```python
from build123d import *

# Parameters (mm, degrees)
SKETCH1_R           = 28.575
BOSS_EXTRUDE1_DEPTH = 22.225
SKETCH3_R           = 11.1125
BOSS_EXTRUDE2_DEPTH = 25.4
SKETCH4_R           = 22.225
CUT_EXTRUDE1_DEPTH  = 12.7
CUT_EXTRUDE2_DEPTH  = 23.225


with BuildPart() as part:
    # Sketch1 → Boss-Extrude1 (new body)
    with BuildSketch(Plane(origin=(0, 0, 0), x_dir=(1, 0, 0), z_dir=(0, 1, 0))):
        with BuildLine():
            Line((-69.85, 0), (69.85, 0))
            ThreePointArc((69.85, 0), (67.980720293, 10.733361765), (62.592988676, 20.202871225))
            ThreePointArc((62.592988676, 20.202871225), (48.540246687, 52.968596396), (54.358983449, 88.142657944))
            ThreePointArc((54.358983449, 88.142657944), (59.032707712, 126.719542875), (39.21125, 160.143031078))
            ThreePointArc((39.21125, 160.143031078), (38.391163038, 161.227624395), (38.1, 162.555822188))
            Line((38.1, 162.555822188), (38.1, 215.9))
            Line((38.1, 215.9), (-38.1, 215.9))
            Line((-38.1, 215.9), (-38.1, 162.555822188))
            ThreePointArc((-38.1, 162.555822188), (-38.391163038, 161.227624395), (-39.21125, 160.143031078))
            ThreePointArc((-39.21125, 160.143031078), (-59.032707712, 126.719542875), (-54.358983449, 88.142657944))
            ThreePointArc((-54.358983449, 88.142657944), (-48.540246687, 52.968596396), (-62.592988676, 20.202871225))
            ThreePointArc((-62.592988676, 20.202871225), (-67.980720293, 10.733361765), (-69.85, 0))
        make_face()
        with Locations((0, 114.3)):
            Circle(SKETCH1_R, mode=Mode.SUBTRACT)
    extrude(amount=BOSS_EXTRUDE1_DEPTH)

    # Sketch3 → Boss-Extrude2 (add)
    with BuildSketch(Plane(origin=(0, 0, -215.9), x_dir=(-1, 0, 0), z_dir=(0, 0, -1))):
        with BuildLine():
            Line((-38.1, 22.225), (38.1, 22.225))
            Line((38.1, 22.225), (38.1, 66.675))
            ThreePointArc((38.1, 66.675), (0, 104.775), (-38.1, 66.675))
            Line((-38.1, 66.675), (-38.1, 22.225))
        make_face()
        with Locations((0, 66.675)):
            Circle(SKETCH3_R, mode=Mode.SUBTRACT)
    extrude(amount=-BOSS_EXTRUDE2_DEPTH)

    # Sketch4 → Cut-Extrude1 (cut)
    with BuildSketch(Plane.XY.offset(-190.5)):
        with Locations((0, 66.675)):
            Circle(SKETCH4_R)
    extrude(amount=-CUT_EXTRUDE1_DEPTH, mode=Mode.SUBTRACT)

    # Sketch5 → Cut-Extrude2 (cut, through all)
    with BuildSketch(Plane(origin=(0, 22.225, 0), x_dir=(1, 0, 0), z_dir=(0, 1, 0))):
        with BuildLine():
            ThreePointArc((39.21125, 160.143031078), (40.964734437, 158.583136265), (42.656216575, 156.956216575))
            Line((42.656216575, 156.956216575), (51.593275336, 165.893275336))
            Line((51.593275336, 165.893275336), (44.768280684, 172.718269988))
            Line((44.768280684, 172.718269988), (38.1, 166.049989304))
            Line((38.1, 166.049989304), (38.1, 162.555822188))
            ThreePointArc((38.1, 162.555822188), (38.391163038, 161.227624395), (39.21125, 160.143031078))
        make_face()
        with BuildLine():
            ThreePointArc((12.193016824, 140.143006128), (16.442699368, 137.670243099), (20.205576272, 134.505576272))
            Line((20.205576272, 134.505576272), (42.656216575, 156.956216575))
            ThreePointArc((42.656216575, 156.956216575), (40.964734437, 158.583136265), (39.21125, 160.143031078))
            ThreePointArc((39.21125, 160.143031078), (38.391163038, 161.227624395), (38.1, 162.555822188))
            Line((38.1, 162.555822188), (38.1, 166.049989304))
            Line((38.1, 166.049989304), (12.193016824, 140.143006128))
        make_face()
        with BuildLine():
            Line((51.593275336, 165.893275336), (42.656216575, 156.956216575))
            ThreePointArc((42.656216575, 156.956216575), (45.942151261, 153.395068263), (48.931671801, 149.581682497))
            Line((48.931671801, 149.581682497), (58.418269988, 159.068280684))
            Line((58.418269988, 159.068280684), (51.593275336, 165.893275336))
        make_face()
        with BuildLine():
            Line((42.656216575, 156.956216575), (20.205576272, 134.505576272))
            ThreePointArc((20.205576272, 134.505576272), (23.370243099, 130.742699368), (25.843006128, 126.493016824))
            Line((25.843006128, 126.493016824), (48.931671801, 149.581682497))
            ThreePointArc((48.931671801, 149.581682497), (45.942151261, 153.395068263), (42.656216575, 156.956216575))
        make_face()
    extrude(amount=-CUT_EXTRUDE2_DEPTH, mode=Mode.SUBTRACT)


solid = part.part
```
Geometry: final body of the model. Coordinates: model frame, mm. A direction names the side the tool comes from. Coordinates: 2 decimals unless noted, no trailing zeros. Write each loop counter-clockwise with the first axis right and the second up, starting at its lowest first coordinate (ties: lowest second). Pieces come first, ordered by that corner, then holes. Notation, with made-up numbers: M 58,17.25 L 70,17.25 A16 cw 70,30.25 Z; hole C 3,30 d1. An arc over 180 degrees is marked long. Use CSV: the item, a comma, the result in double quotes. Start each with the question number.
1. First-contact query: P1, Ø4, axis at y = 23, z = -54.5, coming from the -X side; P2, Ø2, axis at y = 24.5, z = -68.5, coming from the -X side; P3, Ø25, axis at y = 38, z = -197, coming from the +X side. Flat tips, straight axial feed; report the tip coordinate or a pass-through.
2. Reachability of faces 1 (the face through (38.1, 26, -197)), 2 (the face through (5, 77, -203.2)), 3 (the face through (-1, 22.225, -75)) from +Z, -Z, +X, -X, +Y, -Y: full face, straight path, thin tool, end or side. Return the list, or none.
3. Cut plane C-C on y = 63.5. Return the cut outline in (x, z).
4. Cut plane D-D on x = 17.5. Return the cut outline in (y, z) (3 decimals).
5. Cut plane A-A on z = -114.3. Return the cut outline in (x, y) (3 decimals).
6. Mould query, pull axis Z, two halves, no side actions, for faces 4 (the face through (-67.929, 10.957, -10.877)), 5 (the face through (25.33, 11.27, -153.28)), 6 (the face through (-7.9, 45.7, -190.5)). Classes: pulls with the +Z half, pulls with the -Z half, needs draft (parallel to the pull), parting line crosses it, or undercut.
7. Ray query, probe 1 along Y at (x, z) = (0, -195) (3 decimals); probe 2 along X at (y, z) = (4.75, -114.3) (3 decimals); probe 3 along Z at (x, y) = (0, 6.25) (3 decimals). Return the intervals inside material, ascending.
8. Cut plane B-B on x = 0. Count the separate pieces of the cut face and the enclosed holes in it, plus the area to 3 significant figures.
Entries:
1,P1,"x = -48.58"
1,P2,"through"
1,P3,"x = 38.1"
2,face 1,"-Z, +X, +Y, -Y"
2,face 2,"+Z"
2,face 3,"+Z, +X, -X, +Y"
3,outline,"M -38.1,-215.9 L -10.65,-215.9 L -10.65,-203.2 L -22,-203.2 L -22,-190.5 L -38.1,-190.5 Z; M 10.65,-215.9 L 38.1,-215.9 L 38.1,-190.5 L 22,-190.5 L 22,-203.2 L 10.65,-203.2 Z"
4,outline,"M 0,-215.9 L 100.518,-215.9 L 100.518,-190.5 L 80.375,-190.5 L 80.375,-203.2 L 52.975,-203.2 L 52.975,-190.5 L 22.225,-190.5 L 22.225,-145.45 L 0,-145.45 Z; M 0,-91.711 L 22.225,-91.711 L 22.225,0 L 0,0 Z"
5,outline,"M -60.325,0 L -28.575,0 L -28.575,22.225 L -60.325,22.225 Z; M 28.575,0 L 60.325,0 L 60.325,22.225 L 28.575,22.225 Z"
6,face 4,"pulls with the -Z half"
6,face 5,"undercut"
6,face 6,"pulls with the +Z half"
7,probe 1,"0 to 44.45, 88.9 to 104.775"
7,probe 2,"-60.325 to -28.575, 28.575 to 60.325"
7,probe 3,"-215.9 to -142.875, -85.725 to 0"
8,separate pieces,"3"
8,enclosed holes,"0"
8,area,"4,780 mm²"
